Part model, mm, in its own coordinate system. A direction names the side the tool comes from. Coordinates: 2 decimals unless noted, no trailing zeros. Write each loop counter-clockwise with the first axis right and the second up, starting at its lowest first coordinate (ties: lowest second). Pieces come first, ordered by that corner, then holes. Notation, with made-up numbers: (-29, -31.5) - (-2, -31.5) arc R5 ccw to (-2, -25.5) - close; hole circle Ø8 at (61, 78). An arc over 180 degrees is marked (long way). Use one line per item in the form item = value. Start each with the question number.
Autodesk Inventor part; units mm, degrees
ref_plane "YZ Plane" through (0, 0, 0) normal (1, 0, 0) x (0, 1, 0)
ref_plane "XZ Plane" through (0, 0, 0) normal (0, 1, 0) x (-1, 0, 0)
ref_plane "XY Plane" through (0, 0, 0) normal (0, 0, 1) x (1, 0, 0)
sketch "Эскиз1" plane through (0, 0, 0) normal (0, 1, 0) x (-1, 0, 0)
  line L0 (70, -35) -> (62.5, -35)
  line L1 (0, -35) -> (7.5, -35)
  circle A0 centre (66, -13) radius 1.5
  circle A1 centre (4, -13) radius 1.5
  line L2 (70, -8) -> (0, -8)
  line L3 (70, -35) -> (70, -8)
  line L4 (0, -35) -> (0, -8)
  arc A2 (62.5, -35) -> (7.5, -35) centre (35, -76.7582) ccw
  point P0 (0, 0)
  dimension "d4" = 7.5
  dimension "d5" = 7.5
  dimension "d7" = 3
  dimension "d8" = 3
  dimension "d12" = 62
  dimension "d13" = 13
  dimension "d46" = 5
  dimension "d48" = 50
extrude "Выдавливание1" add sketch "Эскиз1" along normal blind 2.5
sketch "Эскиз2" plane through (0, 2.5, 0) normal (0, 1, 0) x (1, 0, 0)
  line L0 (-55, 27) -> (-47.5, 27)
  line L1 (-47.5, 27) -> (-47.5, 17)
  line L2 (-47.5, 17) -> (-55, 17)
  line L3 (-55, 17) -> (-55, 27)
  line L4 (-22.5, 27) -> (-15, 27)
  line L5 (-15, 27) -> (-15, 17)
  line L6 (-15, 17) -> (-22.5, 17)
  line L7 (-22.5, 17) -> (-22.5, 27)
  line L8 (-70, 35) -> (-70, 8)
  line L9 (0, 8) -> (0, 35)
  point P0 (0, 0)
  point P1 (-60, 0)
  point P2 (-15, 22)
  dimension "d17" = 7.5
  dimension "d18" = 10
  dimension "d19" = 7.5
  dimension "d20" = 10
  dimension "d23" = 17
  dimension "d24" = 17
  dimension "d49" = 15
  dimension "d50" = 15
extrude "Выдавливание2" add sketch "Эскиз2" along normal blind 30
sketch "Эскиз3" plane through (-55, 2.5, -27) normal (-1, 0, 0) x (0, 0, 1)
  line L0 (2.15, 27.5) -> (7.85, 27.5)
  line L1 (7.85, 27.5) -> (7.85, 24.9)
  line L2 (7.85, 24.9) -> (2.15, 24.9)
  line L3 (2.15, 24.9) -> (2.15, 27.5)
  line L4 (10, 0) -> (10, 30)
  line L5 (0, 30) -> (10, 30)
  circle A0 centre (5, 22) radius 2.2
  point P0 (27, -2.5)
  dimension "d27" = 5.7
  dimension "d28" = 2.15
  dimension "d29" = 2.6
  dimension "d30" = 2.5
  dimension "d31" = 4.4
  dimension "d32" = 8
  dimension "d44" = 5
extrude "Выдавливание3" cut sketch "Эскиз3" against normal blind 41
sketch "Эскиз4" plane through (0, 32.5, 0) normal (0, 1, 0) x (1, 0, 0)
  circle A0 centre (-18.75, 22) radius 1.6
  circle A1 centre (-51.25, 22) radius 1.6
  line L0 (-22.5, 27) -> (-22.5, 17)
  line L1 (-22.5, 17) -> (-15, 17)
  line L2 (-55, 17) -> (-47.5, 17)
  line L3 (-55, 27) -> (-55, 17)
  point P0 (0, 0)
  point P1 (-18.75, 17)
  dimension "d35" = 3.2
  dimension "d36" = 3.2
  dimension "d37" = 3.75
  dimension "d38" = 5
  dimension "d39" = 5
  dimension "d40" = 3.75
extrude "Выдавливание4" cut sketch "Эскиз4" against normal blind 8
fillet "Сопряжение2" radius 2 8 edges at (-15, 17.5, -27) (-15, 17.5, -17) (-22.5, 17.5, -27) (-22.5, 17.5, -17) (-55, 17.5, -27) (-47.5, 17.5, -27) (-55, 17.5, -17) (-47.5, 17.5, -17)
properties part number "kreplenie_dribler_V2"
Q1. Pin check, flat tips, straight feed: P1, Ø2, axis at y = 19.5, z = -20, coming from the -X side; P2, Ø3, axis at x = -19, y = 19.5, coming from the +Z side; P3, Ø4, axis at y = 17.5, z = -30.5, coming from the +X side; P4, Ø12, axis at y = 27.5, z = -29.5, coming from the +X side. Stop position of each tip, or through.
Q2. Slice it at B-B (z = -13). List the corners of the cut face in (x, y).
Q3. Slice it at C-C (x = -4). List the corners of the cut face in (y, z), plus the area to 3 significant figures.
Q4. Mould opens along Z. For faces 5 (the flat face through (-35, 2.5, -18)), 6 (the flat face through (-51, 29, -24.85)), 7 (the cylindrical face through (-15.57, 17.71, -26.4)) say: released by +Z, released by -Z, zero draft, split by the parting line, or undercut.
Q5. Slice it at D-D (x = -48.5). List the corners of the cut face in (y, z).
Q6. Drill centre lines: probe 1 along X at (y, z) = (26.9, -22); probe 2 along Z at (x, y) = (-51.25, 31.6); probe 3 along X at (y, z) = (7.5, -21.5). Where is each one in solid material? Low to high.
Q7. Slice it at A-A (y = 7.5). List the corners of the cut face in (x, z), plus the area to 3 significant figures.
Q8. Which spindle directions (+Z, -Z, +X, -X, +Y, -Y) get a long thin tool onto all of the face, cutting with end or side? Do faces 1 (the flat face through (-19, 29, -19.15)), 2 (the flat face through (-19, 17, -27)), 3 (the cylindrical face through (-48.1, 17.71, -17.57)), 4 (the cylindrical face through (-15.6, 17.71, -17.57)). Say none if no direction does.
Solution:
q1.P1 = -55
q1.P2 = -17
q1.P3 = through
q1.P4 = -15
q2.outline = (-70, 0) - (-67.5, 0) - (-67.5, 2.5) - (-70, 2.5) - close; (-64.5, 0) - (-5.5, 0) - (-5.5, 2.5) - (-64.5, 2.5) - close; (-2.5, 0) - (0, 0) - (0, 2.5) - (-2.5, 2.5) - close
q3.outline = (0, -35) - (2.5, -35) - (2.5, -14.5) - (0, -14.5) - close; (0, -11.5) - (2.5, -11.5) - (2.5, -8) - (0, -8) - close
q3.area = 60.0 mm2
q4.face_5 = zero draft
q4.face_6 = undercut
q4.face_7 = released by -Z
q5.outline = (0, -28.62) - (2.5, -28.62) - (2.5, -26.73) - (32.5, -26.73) - (32.5, -17.27) - (2.5, -17.27) - (2.5, -8) - (0, -8) - close; hole circle Ø4.4 at (24.5, -22); hole (27.4, -24.85) - (30, -24.85) - (30, -19.15) - (27.4, -19.15) - close
q6.probe_1 = -55 to -52.85, -49.65 to -47.5, -22.5 to -20.35, -17.15 to -15
q6.probe_2 = -27 to -23.6, -20.4 to -17
q6.probe_3 = -55 to -47.5, -22.5 to -15
q7.outline = (-55, -25) arc R2 ccw to (-53, -27) - (-49.5, -27) arc R2 ccw to (-47.5, -25) - (-47.5, -19) arc R2 ccw to (-49.5, -17) - (-53, -17) arc R2 ccw to (-55, -19) - close; (-22.5, -25) arc R2 ccw to (-20.5, -27) - (-17, -27) arc R2 ccw to (-15, -25) - (-15, -19) arc R2 ccw to (-17, -17) - (-20.5, -17) arc R2 ccw to (-22.5, -19) - close
q7.area = 143 mm2
q8.face_1 = +X, -X
q8.face_2 = -Z, +X, -X, +Y
q8.face_3 = +Z, +Y
q8.face_4 = +Z, +X, +Y
